Source: CAD feature listing. Evaluate the final solid. Frame: model axes, mm. A direction names the side the tool comes from. Give positions to 0.01 mm unless a question says otherwise; leave off trailing zeros. Loops run counter-clockwise (first coordinate to the right, second up) from the corner with the lowest first, then second, coordinate; pieces in that order, holes last. Notation, with made-up numbers: M -21.5,-30.5 L 12.5,-30.5 A19 cw 12.5,-21.5 Z; hole C -2.75,87 d5. An arc over 180 degrees is marked long. Put each result on its own line as item: value.
from build123d import *

# Parameters (mm, degrees)
SKETCH1_W                           = 66.04
SKETCH1_H                           = 84.836
BOSS_EXTRUDE1_DEPTH                 = 2.54
F_7_32_0_21875_DIAMETER_SLOT1_DEPTH = 2.54
SKETCH4_W                           = 66.04
SKETCH4_H                           = 38.1
BOSS_EXTRUDE2_DEPTH                 = 55.245
BOSS_EXTRUDE3_DEPTH                 = 34.7218
BOSS_EXTRUDE4_DEPTH                 = 20.3962


# Read off the part's stored shape, not the designer's step: 7/32 (0.21875) Diameter Slot1
with BuildPart() as part:
    # Sketch1 → Boss-Extrude1 (new body)
    with BuildSketch(Plane(origin=(0, 0, 0), x_dir=(1, 0, 0), z_dir=(0, 1, 0))):
        Rectangle(SKETCH1_W, SKETCH1_H)
    extrude(amount=BOSS_EXTRUDE1_DEPTH)

    # 7/32 (0.21875) Diameter Slot1 outline → 7/32 (0.21875) Diameter Slot1 (cut)
    with BuildSketch(Plane(origin=(0, 0, 0), x_dir=(1, 0, 0), z_dir=(0, 1, 0))):
        with BuildLine():
            Line((-24.272875, -36.337875), (-24.272875, -30.718125))
            ThreePointArc((-24.272875, -30.718125), (-27.051, -27.94), (-29.829125, -30.718125))
            Line((-29.829125, -30.718125), (-29.829125, -36.337875))
            ThreePointArc((-29.829125, -36.337875), (-27.051, -39.116), (-24.272875, -36.337875))
        make_face()
        with BuildLine():
            ThreePointArc((-24.272875, 36.337875), (-27.051, 39.116), (-29.829125, 36.337875))
            Line((-29.829125, 36.337875), (-29.829125, 30.718125))
            ThreePointArc((-29.829125, 30.718125), (-27.051, 27.94), (-24.272875, 30.718125))
            Line((-24.272875, 30.718125), (-24.272875, 36.337875))
        make_face()
        with BuildLine():
            Line((29.829125, -36.337875), (29.829125, -30.718125))
            ThreePointArc((29.829125, -30.718125), (27.051, -27.94), (24.272875, -30.718125))
            Line((24.272875, -30.718125), (24.272875, -36.337875))
            ThreePointArc((24.272875, -36.337875), (27.051, -39.116), (29.829125, -36.337875))
        make_face()
        with BuildLine():
            ThreePointArc((29.829125, 36.337875), (27.051, 39.116), (24.272875, 36.337875))
            Line((24.272875, 36.337875), (24.272875, 30.718125))
            ThreePointArc((24.272875, 30.718125), (27.051, 27.94), (29.829125, 30.718125))
            Line((29.829125, 30.718125), (29.829125, 36.337875))
        make_face()
    extrude(amount=F_7_32_0_21875_DIAMETER_SLOT1_DEPTH, mode=Mode.SUBTRACT)

    # Sketch4 → Boss-Extrude2 (add)
    with BuildSketch(Plane(origin=(0, 2.54, 0), x_dir=(1, 0, 0), z_dir=(0, 1, 0))):
        Rectangle(SKETCH4_W, SKETCH4_H)
    extrude(amount=BOSS_EXTRUDE2_DEPTH)

    # Sketch5 → Boss-Extrude3 (add)
    with BuildSketch(Plane(origin=(0, 11.43, 0), x_dir=(1, 0, 0), z_dir=(0, 1, 0))):
        with BuildLine():
            Line((-21.59, 15.748), (-21.59, -15.748))
            ThreePointArc((-21.59, -15.748), (-17.870256121, -24.728256121), (-8.89, -28.448))
            Line((-8.89, -28.448), (8.89, -28.448))
            ThreePointArc((8.89, -28.448), (17.870256121, -24.728256121), (21.59, -15.748))
            Line((21.59, -15.748), (21.59, 15.748))
            ThreePointArc((21.59, 15.748), (17.870256121, 24.728256121), (8.89, 28.448))
            Line((8.89, 28.448), (-8.89, 28.448))
            ThreePointArc((-8.89, 28.448), (-17.870256121, 24.728256121), (-21.59, 15.748))
        make_face()
    extrude(amount=BOSS_EXTRUDE3_DEPTH)

    # Sketch6 → Boss-Extrude4 (add)
    with BuildSketch(Plane(origin=(0, 46.1518, 0), x_dir=(1, 0, 0), z_dir=(0, 1, 0))):
        Polygon((22.86, -19.05), (-22.86, -19.05), (-22.86, -49.53), (-21.336, -49.53), (-21.336, -28.448), (-11.811, -28.448), (-11.811, -49.53), (-10.287, -49.53), (-10.287, -28.448), (-0.762, -28.448), (-0.762, -49.53), (0.762, -49.53), (0.762, -28.448), (10.287, -28.448), (10.287, -49.53), (11.811, -49.53), (11.811, -28.448), (21.336, -28.448), (21.336, -49.53), (22.86, -49.53), align=None)
    boss_extrude4 = extrude(amount=BOSS_EXTRUDE4_DEPTH)

    # Mirror1: Boss-Extrude4 across plane
    add(boss_extrude4.mirror(Plane.XY))


solid = part.part
1. Section query D-D (y = 26). Output: boundary loops of the cut face in (x, z).
Found:
outline: M -33.02,-19.05 L -21.15,-19.05 A12.7 ccw -8.89,-28.45 L 8.89,-28.45 A12.7 ccw 21.15,-19.05 L 33.02,-19.05 L 33.02,19.05 L 21.15,19.05 A12.7 ccw 8.89,28.45 L -8.89,28.45 A12.7 ccw -21.15,19.05 L -33.02,19.05 Z
2. Draft query along Z for faces 5 (the flat face through (-33.02, 28, 1)), 6 (the flat face through (-24.273, 1, -33)), 7 (the cylindrical face through (-16.707, 28.548, 25.757)). Return one class per face: pulls with the +Z half, pulls with the -Z half, needs draft (parallel to the pull), parting line crosses it, or undercut.
Found:
face 5: needs draft
face 6: undercut
face 7: pulls with the +Z half
3. Contact query for flat-ended pins moving along their axis: P1, Ø6, axis at y = 55, z = 32.5, coming from the -X side; P2, Ø2, axis at x = -3, y = 1, coming from the -Z side; P3, Ø6, axis at y = 54.5, z = 43.5, coming from the +X side; P4, Ø12, axis at y = 9, z = -39, coming from the -X side. Output: stop coordinate, or through.
Found:
P1: x = -22.86
P2: z = -42.42
P3: x = 22.86
P4: through
4. Section query C-C (z = 23.5). Output: boundary loops of the cut face in (x, y).
Found:
outline: M -33.02,0 L 33.02,0 L 33.02,2.54 L -33.02,2.54 Z; M -22.86,46.15 L -18.95,46.15 L -18.95,11.43 L 18.95,11.43 L 18.95,46.15 L 22.86,46.15 L 22.86,66.55 L -22.86,66.55 Z
5. Material intervals for line 1 (Y direction, x = -0.5, z = -29); line 2 (Y direction, x = 12, z = -34.5); line 3 (Z direction, x = -13, y = 4), sorted ascending. Write a range as from..to.
Found:
line 1: 0..2.54, 46.15..66.55
line 2: 0..2.54
line 3: -19.05..19.05
6. Section query A-A (z = 40.5). Output: boundary loops of the cut face in (x, y).
Found:
outline: M -33.02,0 L 33.02,0 L 33.02,2.54 L -33.02,2.54 Z; M -22.86,46.15 L -21.34,46.15 L -21.34,66.55 L -22.86,66.55 Z; M -11.81,46.15 L -10.29,46.15 L -10.29,66.55 L -11.81,66.55 Z; M -0.76,46.15 L 0.76,46.15 L 0.76,66.55 L -0.76,66.55 Z; M 10.29,46.15 L 11.81,46.15 L 11.81,66.55 L 10.29,66.55 Z; M 21.34,46.15 L 22.86,46.15 L 22.86,66.55 L 21.34,66.55 Z
7. Section query B-B (x = -27.5). Output: boundary loops of the cut face in (y, z) (3 decimals).
Found:
outline: M 0,-42.418 L 2.54,-42.418 L 2.54,-39.079 L 0,-39.079 Z; M 0,-27.977 L 2.54,-27.977 L 2.54,-19.05 L 57.785,-19.05 L 57.785,19.05 L 2.54,19.05 L 2.54,27.977 L 0,27.977 Z; M 0,39.079 L 2.54,39.079 L 2.54,42.418 L 0,42.418 Z
8. Access query for faces 1 (the flat face through (-21.336, 56, -39)), 2 (the flat face through (22.86, 56, 35)), 3 (the flat face through (0, 11.43, -24)), 4 (the flat face through (-29.829, 1, 33)). Directions: +Z, -Z, +X, -X, +Y, -Y. A direction counts if a zero-diameter tool reaches every point of the face in a straight line with its end or side. Return the directions, or none.
Found:
face 1: -Z, +Y
face 2: +Z, +X, +Y
face 3: -Z, +X, -X
face 4: +Y, -Y
